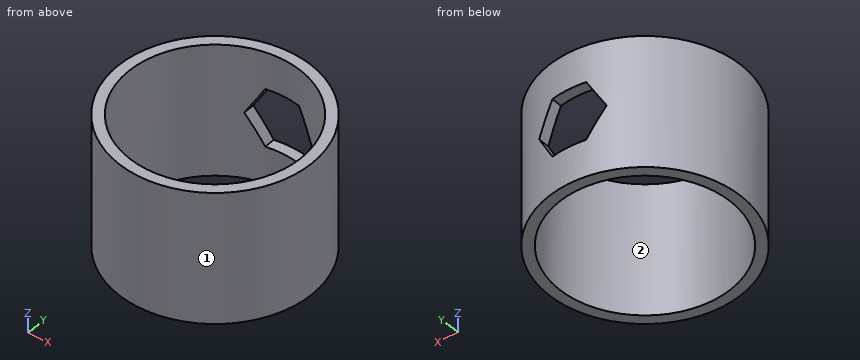
```python
from build123d import *

# Parameters (mm, degrees)
F0_R     = 36.5
F0_R_2   = 32.5
F1_DEPTH = 25
F3_DEPTH = 40


# Not quite as in the source:
# - a feature names something its author has since deleted; it is built from what else it names


with BuildPart() as f1:
    # F0 (on Top) → F1 (new body, symmetric)
    with BuildSketch(Plane.XY):
        Circle(F0_R)
        Circle(F0_R_2, mode=Mode.SUBTRACT)
    extrude(amount=F1_DEPTH, both=True)

    # F2 (on Front) → F3 (cut)
    with BuildSketch(Plane.XZ):
        Polygon((-6.3508529611, -11), (6.3508529611, -11), (12.7017059222, 0), (6.3508529611, 11), (-6.3508529611, 11), (-12.7017059222, 0), align=None)
    extrude(amount=-F3_DEPTH, mode=Mode.SUBTRACT)


solid = f1.part
```
Model file for the job. Use its own axes, mm. Face numbers are marked on the shaded views. Coordinates: 2 decimals unless noted, no trailing zeros. Order: outer loops, then holes, each group sorted by start corner. A loop starts at its lowest first (then second) coordinate and runs counter-clockwise, first axis right, second up. Notation, with made-up numbers: (-29, 49) - (-6, 49) arc R22 cw to (-6, 82) - close; hole circle Ø8 at (-38.5, 25). An arc over 180 degrees is marked (long way). Return JSON: item names as keys, results as strings. Group by question number.
1) Saw through at C-C, the plane x = 0. Write the cut outline in (y, z), plus the area to 3 significant figures.
2) Saw through at A-A, the plane y = 0. Write the cut outline in (x, z), plus the area to 3 significant figures.
3) Saw through at B-B, the plane x = 26.5. Write the cut outline in (y, z).
4) Flat gauge pins, fed straight in: P1, Ø1, axis at x = -24, z = 2.5, coming from the -Y side; P2, Ø8, axis at y = 17.5, z = -7.5, coming from the +X side; P3, Ø3, axis at y = 11, z = 0, coming from the +X side. Where does each tip first touch, or does it go through?
5) Mould opens along Y. For the marked faces 1 and 2 say: released by +Y, released by -Y, zero draft, split by the parting line, or undercut.
6) Probe line 1 (Y direction, x = 1, z = 21); line 2 (Y direction, x = 0, z = 5); line 3 (Y direction, x = -30, z = 16). List the from-to ranges inside material, lowest first. Write a range as from..to.
7) Saw through at D-D, the plane z = 18. Write the cut outline in (x, y).
Values found:
{
 "1": {"outline": "(-36.5, -25) - (-32.5, -25) - (-32.5, 25) - (-36.5, 25) - close; (32.5, -25) - (36.5, -25) - (36.5, -11) - (32.5, -11) - close; (32.5, 11) - (36.5, 11) - (36.5, 25) - (32.5, 25) - close", "area": "312 mm²"},
 "2": {"outline": "(-36.5, -25) - (-32.5, -25) - (-32.5, 25) - (-36.5, 25) - close; (32.5, -25) - (36.5, -25) - (36.5, 25) - (32.5, 25) - close", "area": "400 mm²"},
 "3": {"outline": "(-25.1, -25) - (-18.81, -25) - (-18.81, 25) - (-25.1, 25) - close; (18.81, -25) - (25.1, -25) - (25.1, 25) - (18.81, 25) - close"},
 "4": {"P1": "stops at y = -27.93", "P2": "stops at x = 33.91", "P3": "stops at x = 35.24"},
 "5": {"face 1": "split by the parting line", "face 2": "undercut"},
 "6": {"line 1": "y = -36.49..-32.48, 32.48..36.49", "line 2": "y = -36.5..-32.5", "line 3": "y = -20.79..-12.5, 12.5..20.79"},
 "7": {"outline": "circle Ø73 at (0, 0); hole circle Ø65 at (0, 0)"}
}
